Autodesk Inventor part; units mm, degrees
ref_plane "YZ Plane" through (0, 0, 0) normal (1, 0, 0) x (0, 1, 0)
ref_plane "XZ Plane" through (0, 0, 0) normal (0, 1, 0) x (-1, 0, 0)
ref_plane "XY Plane" through (0, 0, 0) normal (0, 0, 1) x (1, 0, 0)
sketch "Skizze1" plane through (0, 0, 0) normal (0, 1, 0) x (-1, 0, 0)
  circle A0 centre (0, 0) radius 100
  dimension "d0" = 200
extrude "Extrusion1" add sketch "Skizze1" along normal blind 10
sketch "Skizze2" plane through (0, 10, 0) normal (0, 1, 0) x (1, 0, 0)
  circle A0 centre (0, 0) radius 100
  circle A1 centre (-87, 0) radius 3.1
  dimension "d3" = 6.2
  dimension "d4" = 87
  dimension "d5" = 200
extrude "Extrusion2" cut sketch "Skizze2" against normal through all contours A1
chamfer "Fasen1" distance 3 angle 45 1 edges at (-90.1, 0, 0)
sketch "Skizze3" plane through (0, 10, 0) normal (0, 1, 0) x (1, 0, 0)
  circle A0 centre (-87, 0) radius 3.1
  circle A1 centre (0, 0) radius 100
  line L0 (-97, -24.3105) -> (-97, 24.3105)
  circle A2 centre (0, 0) radius 100
  point P0 (-97, -24.3105)
  dimension "d11" = 10
extrude "Extrusion3" cut sketch "Skizze3" against normal through all contours L0 A1 picked at (-97.7491, 4.0825)
pattern_circular "Runde Anordnung3" count 4 over 360 about axis through (0, -10, 0) along (0, 1, 0) of "Extrusion2", "Fasen1"
pattern_circular "Runde Anordnung4" count 4 over 360 about axis through (0, -10, 0) along (0, 1, 0) of "Extrusion3"
sketch "Skizze4" plane through (0, 0, 0) normal (0, -1, 0) x (1, 0, 0)
  circle A0 centre (0, 0) radius 8
  dimension "d26" = 16
extrude "Extrusion4" cut sketch "Skizze4" against normal through all
sketch "Skizze5" plane through (0, 0, 0) normal (0, -1, 0) x (1, 0, 0)
  circle A0 centre (0, 0) radius 8
  circle A1 centre (0, -87) radius 6.1
  circle A2 centre (0, 87) radius 6.1
  line L0 (-24.3105, -97) -> (24.3105, -97)
  arc A3 (24.3105, -97) -> (97, -24.3105) centre (0, 0) ccw
  line L1 (97, -24.3105) -> (97, 24.3105)
  arc A4 (97, 24.3105) -> (24.3105, 97) centre (0, 0) ccw
  line L2 (24.3105, 97) -> (-24.3105, 97)
  arc A5 (-24.3105, 97) -> (-97, 24.3105) centre (0, 0) ccw
  line L3 (-97, 24.3105) -> (-97, -24.3105)
  arc A6 (-97, -24.3105) -> (-24.3105, -97) centre (0, 0) ccw
  circle A7 centre (-87, 0) radius 6.1
  circle A8 centre (87, 0) radius 6.1
  line L4 (-10.25, 76.75) -> (10.25, 76.75)
  line L5 (10.25, 76.75) -> (10.25, 97.25)
  line L6 (10.25, 97.25) -> (-10.25, 97.25)
  line L7 (-10.25, 97.25) -> (-10.25, 76.75)
  line L8 (-10.25, 76.75) -> (10.25, 97.25) construction
  line L9 (10.25, 76.75) -> (-10.25, 97.25) construction
  point P0 (10.25, 97)
  point P1 (-10.25, 97)
  dimension "d29" = 20.5
  dimension "d30" = 20.5
extrude "Extrusion5" cut sketch "Skizze5" against normal through all contours A2 | L2 L5 L4 L7
pattern_circular "Runde Anordnung5" count 4 over 360 about axis through (0, 0, 0) along (0, 1, 0) of "Extrusion5"
sketch "Skizze6" plane through (0, 0, 0) normal (0, -1, 0) x (1, 0, 0)
  line L0 (0, 0) -> (51.2757, 51.2757) construction
  circle A0 centre (0, 0) radius 8
  line L1 (0, 0) -> (0, 40.1538) construction
  circle A1 centre (31.8198, 31.8198) radius 6
  line L2 (0, 0) -> (-46.8461, -46.8461) construction
  circle A2 centre (-31.8198, -31.8198) radius 6
  dimension "d36" = 45
  dimension "d37" = 12
  dimension "d38" = 45
  dimension "d39" = 12
  dimension "d40" = 45
extrude "Extrusion6" cut sketch "Skizze6" against normal through all contours A1 | A2
properties part number "plate_lower"
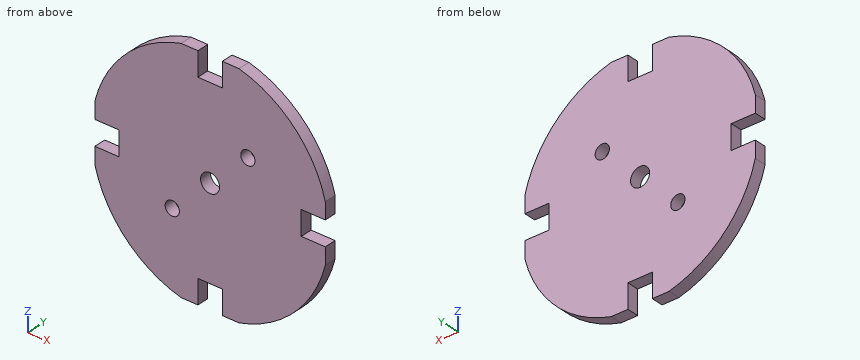
Read the model definition and answer for the solid it produces. Units are mm, in the model's axes. Coordinates: 2 decimals unless noted, no trailing zeros. Loops run counter-clockwise (first coordinate to the right, second up) from the corner with the lowest first, then second, coordinate; pieces in that order, holes last. Notation, with made-up numbers: (75.5, 50.25) -> (109.5, 50.25) arc R25 ccw to (109.5, 63.25) -> close; hole circle Ø10 at (53, -23.75). An arc over 180 degrees is marked (long way). Answer in a Markdown table with one row per item.
Item 1: A cutting plane is placed at B-B on z = 0. Determine the outline of the cut face in (x, y).
Returned:
| item | result |
|---|---|
| outline | (-76.75, 0) -> (-8, 0) -> (-8, 10) -> (-76.75, 10) -> close; (8, 0) -> (76.75, 0) -> (76.75, 10) -> (8, 10) -> close |
Item 2: A cutting plane is placed at A-A on x = 0. Determine the outline of the cut face in (y, z).
Returned:
| item | result |
|---|---|
| outline | (0, -76.75) -> (10, -76.75) -> (10, -8) -> (0, -8) -> close; (0, 8) -> (10, 8) -> (10, 76.75) -> (0, 76.75) -> close |
Item 3: A cutting plane is placed at C-C on y = 1.5. Determine the outline of the cut face in (x, z), plus the area to 3 significant figures.
Returned:
| item | result |
|---|---|
| outline | (-97, -24.31) arc R100 ccw to (-24.31, -97) -> (-10.25, -97) -> (-10.25, -76.75) -> (10.25, -76.75) -> (10.25, -97) -> (24.31, -97) arc R100 ccw to (97, -24.31) -> (97, -10.25) -> (76.75, -10.25) -> (76.75, 10.25) -> (97, 10.25) -> (97, 24.31) arc R100 ccw to (24.31, 97) -> (10.25, 97) -> (10.25, 76.75) -> (-10.25, 76.75) -> (-10.25, 97) -> (-24.31, 97) arc R100 ccw to (-97, 24.31) -> (-97, 10.25) -> (-76.75, 10.25) -> (-76.75, -10.25) -> (-97, -10.25) -> close; hole circle Ø12 at (-31.82, -31.82); hole circle Ø16 at (0, 0); hole circle Ø12 at (31.82, 31.82) |
| area | 28,900 mm^2 |
Item 4: Each of these flat-tipped pins is pushed along its axis until it touches: P1, Ø3, axis at y = 4.5, z = 34.5, coming from the -X side; P2, Ø9.5, axis at x = -31.82, z = -31.82, coming from the -Y side; P3, Ø2, axis at y = 3, z = -77, coming from the +X side; P4, Ø5, axis at x = 5, y = 4.5, coming from the -Z side. Where does it stop, or does it pass through?
Returned:
| item | result |
|---|---|
| P1 | stops at x = -94.4 |
| P2 | passes through |
| P3 | stops at x = 64.99 |
| P4 | stops at z = -76.75 |
Item 5: Straight lines are drawn through the part: line 1 along Z through (x, y) = (0, 8.25); line 2 along X through (y, z) = (6.25, 34.5); line 3 along Z through (x, y) = (27, 2.5). For each, find the intervals that lie inside material, in ascending order. Write a range as [from, to].
Returned:
| item | result |
|---|---|
| line 1 | z = [-76.75, -8], [8, 76.75] |
| line 2 | x = [-93.86, 26.45], [37.19, 93.86] |
| line 3 | z = [-96.29, 28.25], [35.39, 96.29] |
Item 6: A cutting plane is placed at D-D on z = 74. Determine the outline of the cut face in (x, y).
Returned:
| item | result |
|---|---|
| outline | (-67.26, 0) -> (67.26, 0) -> (67.26, 10) -> (-67.26, 10) -> close |
